Autodesk Inventor part; units mm, degrees
ref_plane "YZ Plane" through (0, 0, 0) normal (1, 0, 0) x (0, 1, 0)
ref_plane "XZ Plane" through (0, 0, 0) normal (0, 1, 0) x (-1, 0, 0)
ref_plane "XY Plane" through (0, 0, 0) normal (0, 0, 1) x (1, 0, 0)
sketch "Sketch1" plane through (0, 0, 0) normal (1, 0, 0) x (0, 1, 0)
  circle A0 centre (0, 0) radius 28.575
  circle A1 centre (0, 0) radius 30.1625
  dimension "d0" = 57.15
  dimension "d1" = 60.325
extrude "Extrusion1" add sketch "Sketch1" along normal blind 25.4
sketch "Sketch2" plane through (25.4, 0, 0) normal (1, 0, 0) x (0, 0, -1)
  circle A0 centre (0, 0) radius 28.575
  circle A1 centre (0, 0) radius 30.1625
extrude "Extrusion2" add sketch "Sketch2" against normal blind 6.35 contours A0 | A1
sketch "Sketch3" plane through (25.4, 0, 0) normal (1, 0, 0) x (0, 0, -1)
  line L0 (13.6642, 26.8899) -> (11.89, -27.7201)
  circle A0 centre (0, 0) radius 30.1625
  dimension "d6" = 54.61
extrude "Extrusion3" cut sketch "Sketch3" against normal through all contours A0 L0 picked at (14.9201, 7.4757)
sketch "Sketch4" plane through (25.4, 0, 0) normal (1, 0, 0) x (0, 0, -1)
  circle A0 centre (0, 0) radius 3.175
  dimension "d9" = 6.35
extrude "Extrusion4" cut sketch "Sketch4" against normal through all
sketch "Sketch5" plane through (25.4, 0, 0) normal (1, 0, 0) x (0, 0, -1)
  circle A0 centre (0, 0) radius 3.175
  circle A1 centre (0, 0) radius 6.35
  dimension "d12" = 6.35
  dimension "d13" = 12.7
extrude "Extrusion5" add sketch "Sketch5" along normal blind 19.05
properties part number "chain stashonary out part"
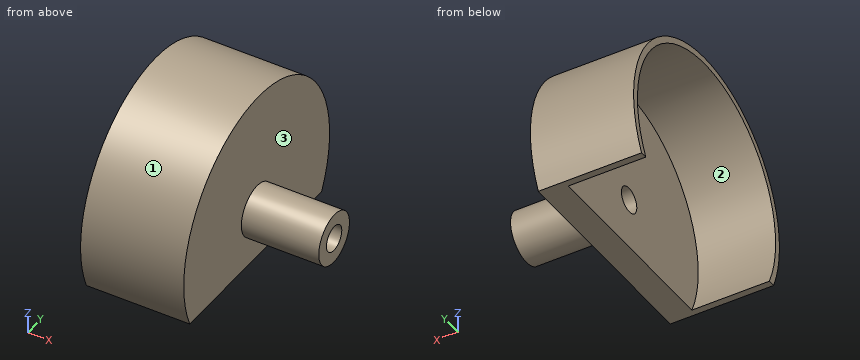
CAD build for the part. Positions are in the model's coordinates, mm. Face numbers are marked on the shaded views. Coordinates: 2 decimals unless noted, no trailing zeros. Write each loop counter-clockwise with the first axis right and the second up, starting at its lowest first coordinate (ties: lowest second). Pieces come first, ordered by that corner, then holes. Notation, with made-up numbers: (-35, -0.5) - (-20, -0.5) arc R26 cw to (-20, 30.5) - close; hole circle Ø5 at (3, -15). An arc over 180 degrees is marked (long way). Use a Markdown table: item, result. Add a question column.
Item 1: Mould opens along Z. For the marked faces 1, 2 and 3 say: pulls with the +Z half, pulls with the -Z half, needs draft (parallel to the pull), parting line crosses it, or undercut.
Item 2: Drill centre lines: L1, parallel to Y at x = 13, z = 0 (1 decimal); L2, parallel to Y at x = 38, z = 0 (3 decimals); L3, parallel to X at y = -9, z = -9.5. Where is each one in solid material? Low to high. Write a range as from..to.
Item 3: Band-saw the part on C-C, the plane z = 8.5. Give the cut face in (x, y).
Item 4: Flat gauge pins, fed straight in: pin 1 (5 mm diameter, centred on y = -12, z = 24.5, fed in from -X); pin 2 (10 mm diameter, centred on x = 38, y = 0.5, fed in from +Z); pin 3 (8.5 mm diameter, centred on y = 0, z = 0, fed in from -X); pin 4 (5 mm diameter, centred on x = 23.5, z = 15.5, fed in from -Y). Where does each tip first touch, or does it go through?
Numbers:
| question | item | result |
|---|---|---|
| 1 | face 1 | parting line crosses it |
| 1 | face 2 | undercut |
| 1 | face 3 | needs draft |
| 2 | L1 | -30.2..-28.6, 28.6..30.2 |
| 2 | L2 | -6.35..-3.175, 3.175..6.35 |
| 2 | L3 | 19.05..25.4 |
| 3 | outline | (0, -28.94) - (25.4, -28.94) - (25.4, 28.94) - (0, 28.94) - (0, 27.28) - (19.05, 27.28) - (19.05, -27.28) - (0, -27.28) - close |
| 4 | pin 1 | x = 0 |
| 4 | pin 2 | z = 6.35 |
| 4 | pin 3 | x = 19.05 |
| 4 | pin 4 | y = -27.22 |
